from build123d import *

# Parameters (mm, degrees)
F1_DEPTH = 25.4
F2_R     = 6.35
F3_DEPTH = 101.601


with BuildPart() as f1:
    # F0 (on Front) → F1 (new body)
    with BuildSketch(Plane.XZ):
        Polygon((-76.2, 22.59441), (-101.6, 22.59441), (-101.6, -28.20559), (-19.05, -28.20559), (-19.05, -15.50559), (0, -15.50559), (0, 22.59441), (-25.4, 22.59441), (-25.4, 12.650757), (-76.2, 12.650757), align=None)
    extrude(amount=F1_DEPTH)

    # F2 (on Right) → F3 (cut, through all)
    with BuildSketch(Plane.YZ):
        with Locations((-12.7, -2.80559)):
            Circle(F2_R)
    extrude(amount=-F3_DEPTH, mode=Mode.SUBTRACT)


solid = f1.part
Check sheet for the modelled part. Datum: model origin and axes. Units: mm. A direction names the side the tool comes from. Round coordinates to 2 decimals unless told otherwise and drop trailing zeros. Order: outer loops, then holes, each group sorted by start corner. A loop starts at its lowest first (then second) coordinate and runs counter-clockwise, first axis right, second up.
(1) Cross-section at C-C, the plane x = -10. Enter the section's corners in (y, z).
(2) Access from +Z, -Z, +X, -X, +Y, -Y to the whole of each face (thin tool, end or side, straight path). Record for faces 5 (the flat face through (-76.2, -13, 18)), 6 (the cylindrical face through (-50.089, -6.643, -0.898)).
(3) Cross-section at B-B, the plane z = -6. Enter the section's corners in (x, y), and give its area (3 significant figures).
(4) Scan lines: probe 1 along Z at (x, y) = (-34, -12.7); probe 2 along Z at (x, y) = (-20.5, -18.5); probe 3 along X at (y, z) = (-17.75, -23.5). Record each from-to range of solid material in increasing order.
(5) Draft check along X on faces 1 (the flat face through (-19.05, -13, -22)), 2 (the flat face through (-25.4, -13, 18)), 3 (the flat face through (-101.6, -15.3, 3.2)), 4 (the flat face through (-10, -13, -15.506)). Enter one of: pulls with the +X half, pulls with the -X half, needs draft (parallel to the pull), parting line crosses it, or undercut.
(6) Cross-section at D-D, the plane z = -20. Enter the section's corners in (x, y), and give its area (3 significant figures).
(7) Cross-section at A-A, the plane y = -12.7. Enter the section's corners in (x, z).
(8) Go/stop test with flat-tipped pins: P1, Ø7.5, axis at x = -42.5, y = -11.5, coming from the +Z side; P2, Ø10, axis at x = -17, z = -7, coming from the +Y side; P3, Ø10, axis at y = -9, z = -22, coming from the +X side; P4, Ø5.5, axis at x = -11, y = -12, coming from the -Z side. Record where each tip stops, or that it passes through.
Check sheet entries:
1. outline: (-25.4, -15.51) - (0, -15.51) - (0, 22.59) - (-25.4, 22.59) - close; hole circle Ø12.7 at (-12.7, -2.81)
2. face 5: +Z, +Y, -Y
2. face 6: +X, -X
3. outline: (-101.6, -25.4) - (0, -25.4) - (0, -18.19) - (-101.6, -18.19) - close; (-101.6, -7.21) - (0, -7.21) - (0, 0) - (-101.6, 0) - close
3. area: 1,470 mm2
4. probe 1: z = -28.21 to -9.16, 3.54 to 12.65
4. probe 2: z = -28.21 to -5.39, -0.22 to 22.59
4. probe 3: x = -101.6 to -19.05
5. face 1: pulls with the +X half
5. face 2: undercut
5. face 3: pulls with the -X half
5. face 4: needs draft
6. outline: (-101.6, -25.4) - (-19.05, -25.4) - (-19.05, 0) - (-101.6, 0) - close
6. area: 2,100 mm2
7. outline: (-101.6, -28.21) - (-19.05, -28.21) - (-19.05, -15.51) - (0, -15.51) - (0, -9.16) - (-101.6, -9.16) - close; (-101.6, 3.54) - (0, 3.54) - (0, 22.59) - (-25.4, 22.59) - (-25.4, 12.65) - (-76.2, 12.65) - (-76.2, 22.59) - (-101.6, 22.59) - close
8. P1: stops at z = 12.65
8. P2: stops at y = 0
8. P3: stops at x = -19.05
8. P4: stops at z = -15.51
